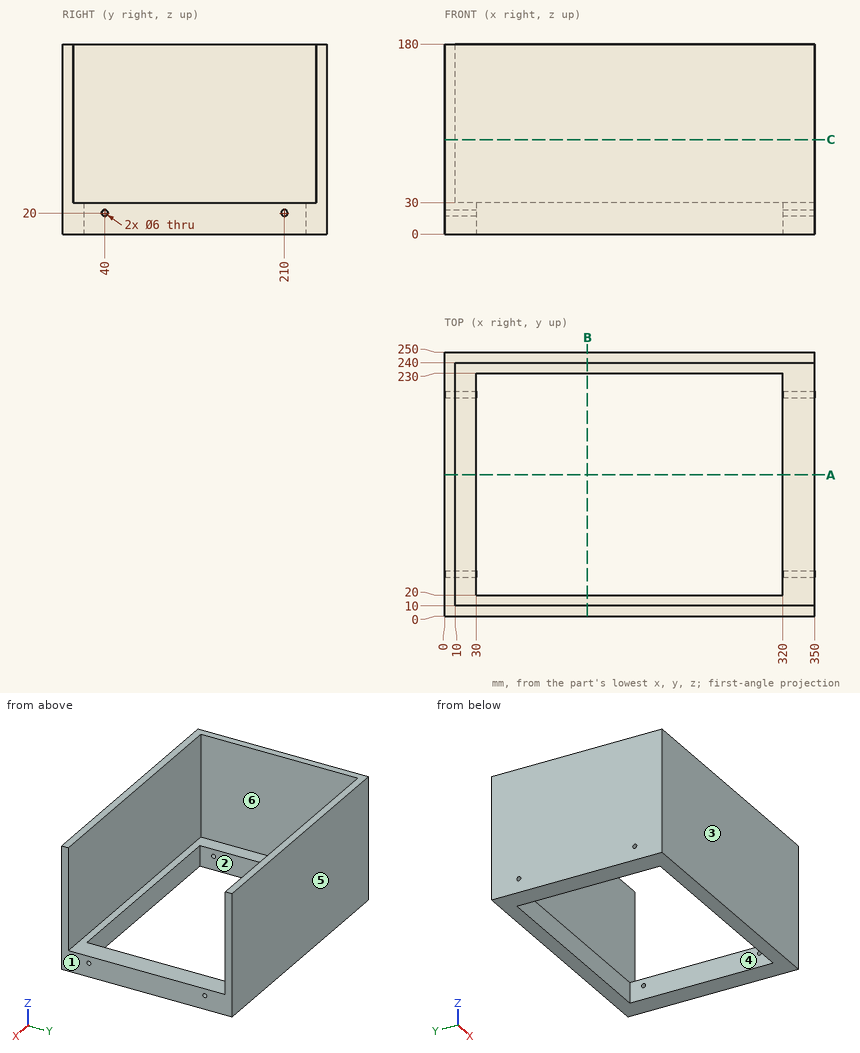
Can you work these out from the drawing? Everything is in mm from the part's minimum corner. A direction names the side the tool comes from. Give positions to 0.01 mm unless a question says otherwise; leave off trailing zeros. Loops run counter-clockwise (first coordinate to the right, second up) from the corner with the lowest first, then second, coordinate; pieces in that order, holes last. Notation, with made-up numbers: M 84,75.5 L 120,75.5 A29 ccw 120,95.5 Z; hole C 55.5,-30 d11. An arc over 180 degrees is marked long. Put each result on its own line as item: value. Start each with the question number.
(1) I want a section at A-A on y = 134. Please give me the cut outline in (x, z).
(2) If we mould it in two halves opening along X, with no side actions, what happens to the marked faces 1, 2 and 3? For each: +X half, -X half, draft (parallel to the pull), parting line (faces both ways), or undercut.
(3) I want a section at B-B on x = 135. Please give me the cut outline in (y, z), then the cut area to 3 significant figures.
(4) Will these pins go through, and if not, where does the flat tip stop? pin 1 Ø3.5 at (y, z) = (40, 20) entering from -X; pin 2 Ø4 at (y, z) = (66, 63) entering from +X.
(5) I want a section at C-C on z = 89.5. Please give me the cut outline in (x, y).
(6) For the marked faces 4, 5 and 6, which set-ups out of +Z, -Z, +X, -X, +Y, -Y let a thin tool reach every point of the face, with its end or its side?
(7) I need wall thicknesses on line 1 along Y through (x, z) = (333.25, 20); line 2 along Y through (x, z) = (91.5, 84.5); line 3 along Z through (x, y) = (7.5, 210). Which ranges of each line are inside material? Lowest first, please. Write a range as [from, to].
Answer block:
1. outline: M 0,0 L 30,0 L 30,30 L 10,30 L 10,180 L 0,180 Z; M 320,0 L 350,0 L 350,30 L 320,30 Z
2. face 1: +X half
2. face 2: undercut
2. face 3: draft
3. outline: M 0,0 L 20,0 L 20,30 L 10,30 L 10,180 L 0,180 Z; M 230,0 L 250,0 L 250,180 L 240,180 L 240,30 L 230,30 Z
3. area: 4,200 mm^2
4. pin 1: through
4. pin 2: x = 10
5. outline: M 0,0 L 350,0 L 350,10 L 10,10 L 10,240 L 350,240 L 350,250 L 0,250 Z
6. face 4: +Z, -Z
6. face 5: +Z, -Z, +X, -X, +Y
6. face 6: +Z, +X
7. line 1: [0, 37], [43, 207], [213, 250]
7. line 2: [0, 10], [240, 250]
7. line 3: [0, 17], [23, 180]
